Verification items for this drawing (mm, ordinates from the low corner). A direction names the side the tool comes from. Give positions to 0.01 mm unless a question says otherwise; leave off trailing zeros. Loops run counter-clockwise (first coordinate to the right, second up) from the corner with the lowest first, then second, coordinate; pieces in that order, holes last. Notation, with made-up numbers: (76.25, 75) -> (117.25, 75) arc R22 ccw to (117.25, 114) -> close; hole circle Ø7 at (61, 59). An arc over 180 degrees is marked (long way). Answer as CSV lines item,"result". Start each with the question number.
(1) Material ranges on line 1 (X direction, y = 4, z = 6.35); line 2 (Z direction, x = 35.56, y = 4.5); line 3 (Y direction, x = 41.91, z = 2), recorded low to high. Write a range as from..to.
(2) Section check D-D on z = 15.24. Enter the section's corners in (x, y).
(3) Release check for a two-part mould opening along X. For the marked faces 3, 4 and 5 record: pulls with the +X half, pulls with the -X half, needs draft (parallel to the pull), parting line crosses it, or undercut.
(4) Section check A-A on x = 41.91. Enter the section's corners in (y, z).
(5) Gauge pin test, flat ends, axial feed: pin 1 Ø5 at (y, z) = (11.5, 15) entering from +X; pin 2 Ø4 at (x, y) = (20, 12) entering from +Z; pin 3 Ø4.5 at (x, z) = (15.5, 8) entering from +Y. Record the tip position at first contact, or that the pin passes through.
(6) Section check B-B on x = 22.86. Enter the section's corners in (y, z).
(7) Access from +Z, -Z, +X, -X, +Y, -Y to the whole of each face (thin tool, end or side, straight path). Record for the marked faces 1 and 2.
(8) Section check C-C on y = 4. Enter the section's corners in (x, z), plus the area to 3 significant figures.
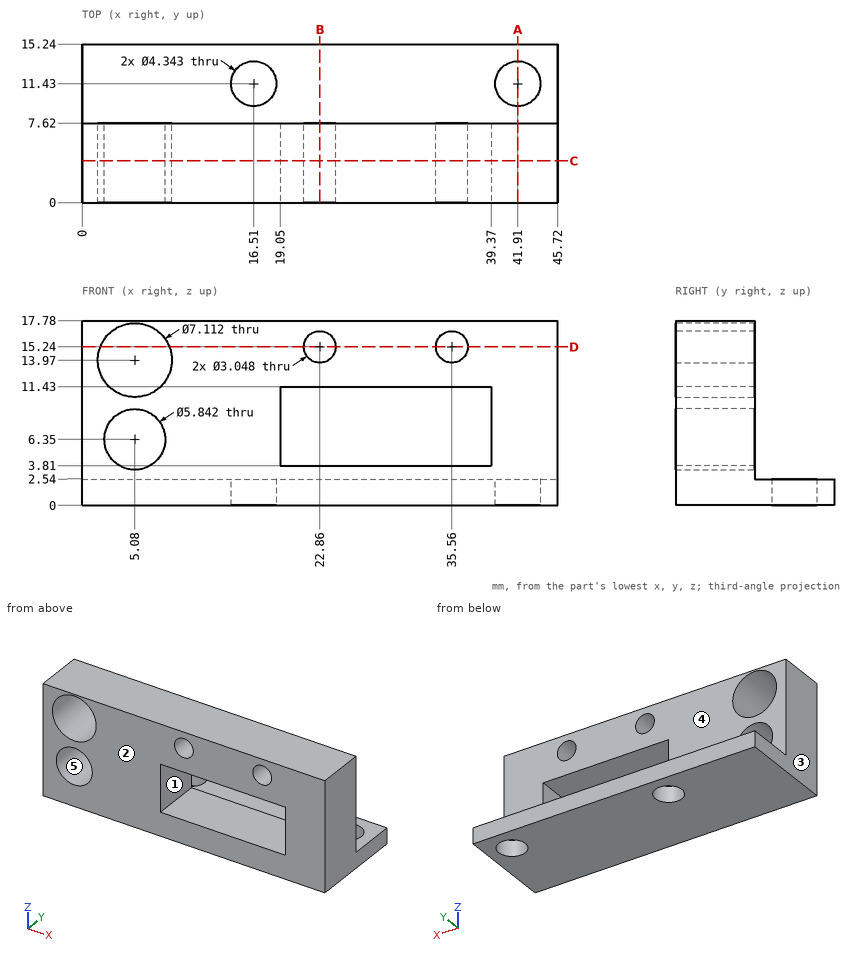
Working result:
1,line 1,"x = 0..2.16, 8..19.05, 39.37..45.72"
1,line 2,"z = 0..3.81, 11.43..13.72, 16.76..17.78"
1,line 3,"y = 0..9.26, 13.6..15.24"
2,outline,"(0, 0) -> (1.76, 0) -> (1.76, 7.62) -> (0, 7.62) -> close; (8.4, 0) -> (21.34, 0) -> (21.34, 7.62) -> (8.4, 7.62) -> close; (24.38, 0) -> (34.04, 0) -> (34.04, 7.62) -> (24.38, 7.62) -> close; (37.08, 0) -> (45.72, 0) -> (45.72, 7.62) -> (37.08, 7.62) -> close"
3,face 3,"pulls with the -X half"
3,face 4,"needs draft"
3,face 5,"undercut"
4,outline,"(0, 0) -> (9.26, 0) -> (9.26, 2.54) -> (7.62, 2.54) -> (7.62, 17.78) -> (0, 17.78) -> close; (13.6, 0) -> (15.24, 0) -> (15.24, 2.54) -> (13.6, 2.54) -> close"
5,pin 1,"passes through"
5,pin 2,"stops at z = 2.54"
5,pin 3,"stops at y = 7.62"
6,outline,"(0, 0) -> (15.24, 0) -> (15.24, 2.54) -> (7.62, 2.54) -> (7.62, 3.81) -> (0, 3.81) -> close; (0, 11.43) -> (7.62, 11.43) -> (7.62, 13.72) -> (0, 13.72) -> close; (0, 16.76) -> (7.62, 16.76) -> (7.62, 17.78) -> (0, 17.78) -> close"
7,face 1,"+Y, -Y"
7,face 2,"+Z, -Z, +X, -X, -Y"
8,outline,"(0, 0) -> (45.72, 0) -> (45.72, 17.78) -> (0, 17.78) -> close; hole circle Ø7.11 at (5.08, 13.97); hole circle Ø5.84 at (5.08, 6.35); hole (19.05, 3.81) -> (39.37, 3.81) -> (39.37, 11.43) -> (19.05, 11.43) -> close; hole circle Ø3.05 at (22.86, 15.24); hole circle Ø3.05 at (35.56, 15.24)"
8,area,"577 mm^2"
